Can you work these out from the drawing? Everything is in mm from the part's minimum corner. A direction names the side the tool comes from. Round coordinates to 2 decimals unless told otherwise and drop trailing zeros. Loops run counter-clockwise (first coordinate to the right, second up) from the corner with the lowest first, then second, coordinate; pieces in that order, holes last. Notation, with made-up numbers: (45.25, -13) -> (89.25, -13) arc R29 cw to (89.25, 10) -> close; hole circle Ø4 at (44.25, -4). An arc over 180 degrees is marked (long way). One line per item, written item: value.
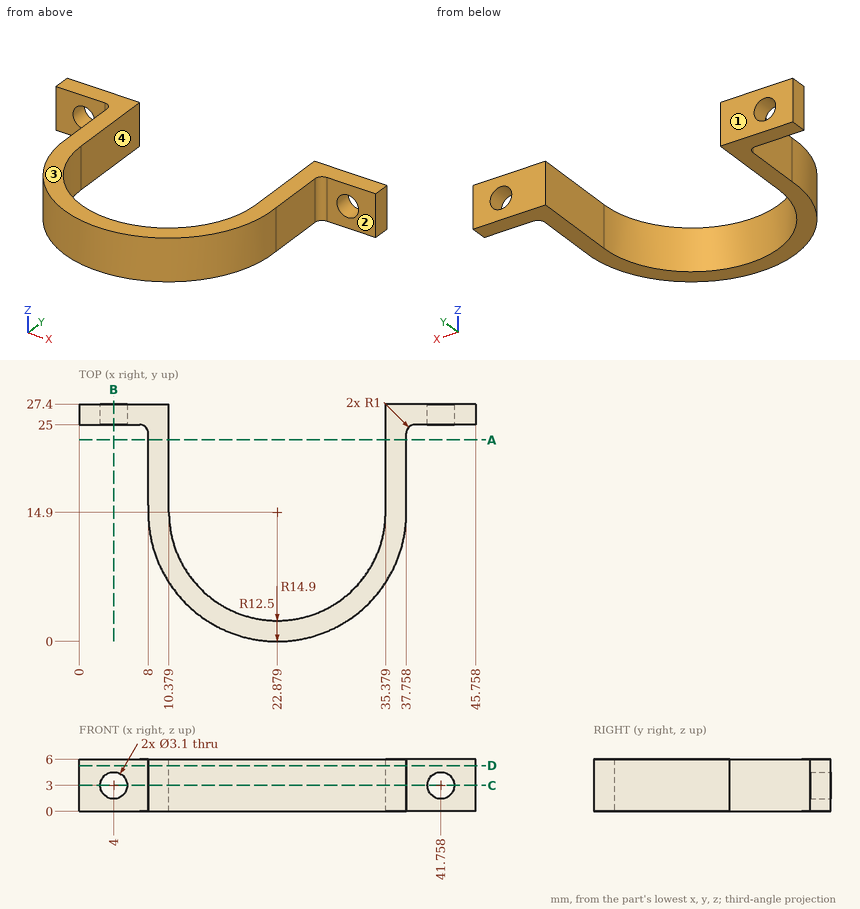
(1) If I drill on L1, parallel to X at y = 26, z = 3; L2, parallel to X at y = 14.5, z = 3.95; L3, parallel to Z at x = 4, y = 26.85, over which ranges is the centre line in solid material (lowest first)?
Recorded:
L1: 0 to 2.45, 5.55 to 10.38, 35.38 to 40.21, 43.31 to 45.76
L2: 7.98 to 10.39, 35.37 to 37.77
L3: 0 to 1.45, 4.55 to 6
(2) I'm going to push flat-ended pins straight in: pin 1 Ø1.8 at (y, z) = (21, 2.5) entering from -X; pin 2 Ø3 at (x, z) = (31, 4.5) entering from +Y. Where does each tip first touch, or does it pass through?
Recorded:
pin 1: x = 8
pin 2: y = 6.92
(3) If we section it at A-A, the plane y = 23.25: Please give me the cut outline in (x, z).
Recorded:
outline: (8, 0) -> (10.38, 0) -> (10.38, 6) -> (8, 6) -> close; (35.38, 0) -> (37.76, 0) -> (37.76, 6) -> (35.38, 6) -> close
(4) If we section it at C-C, the plane z = 3: Please give me the cut outline in (x, y), then the cut area to 3 significant figures.
Recorded:
outline: (0, 25) -> (2.45, 25) -> (2.45, 27.4) -> (0, 27.4) -> close; (5.55, 25) -> (7, 25) arc R1 cw to (8, 24) -> (8, 15.69) arc R14.9 ccw (long way) to (37.76, 15.69) -> (37.76, 24) arc R1 cw to (38.76, 25) -> (40.21, 25) -> (40.21, 27.4) -> (35.38, 27.4) -> (35.38, 14.9) arc R12.5 cw to (10.38, 14.9) -> (10.38, 27.4) -> (5.55, 27.4) -> close; (43.31, 25) -> (45.76, 25) -> (45.76, 27.4) -> (43.31, 27.4) -> close
area: 187 mm²
(5) For the marked faces 1, 2, 3 and 4, which set-ups out of +Z, -Z, +X, -X, +Y, -Y let a thin tool reach every point of the face, with its end or its side?
Recorded:
face 1: +Z, -Z, +X, -X, +Y
face 2: +Z, -Z, +X, -Y
face 3: +Z, +X, -X, +Y, -Y
face 4: +Z, -Z, +Y
(6) If we section it at D-D, the plane z = 5.3: Please give me the cut outline in (x, y), then the cut area to 3 significant figures.
Recorded:
outline: (0, 25) -> (7, 25) arc R1 cw to (8, 24) -> (8, 15.69) arc R14.9 ccw (long way) to (37.76, 15.69) -> (37.76, 24) arc R1 cw to (38.76, 25) -> (45.76, 25) -> (45.76, 27.4) -> (35.38, 27.4) -> (35.38, 14.9) arc R12.5 cw to (10.38, 14.9) -> (10.38, 27.4) -> (0, 27.4) -> close
area: 202 mm²
(7) If we section it at B-B, the plane x = 4: Please give me the cut outline in (y, z), then the cut area to 3 significant figures.
Recorded:
outline: (25, 0) -> (27.4, 0) -> (27.4, 1.45) -> (25, 1.45) -> close; (25, 4.55) -> (27.4, 4.55) -> (27.4, 6) -> (25, 6) -> close
area: 6.96 mm²
